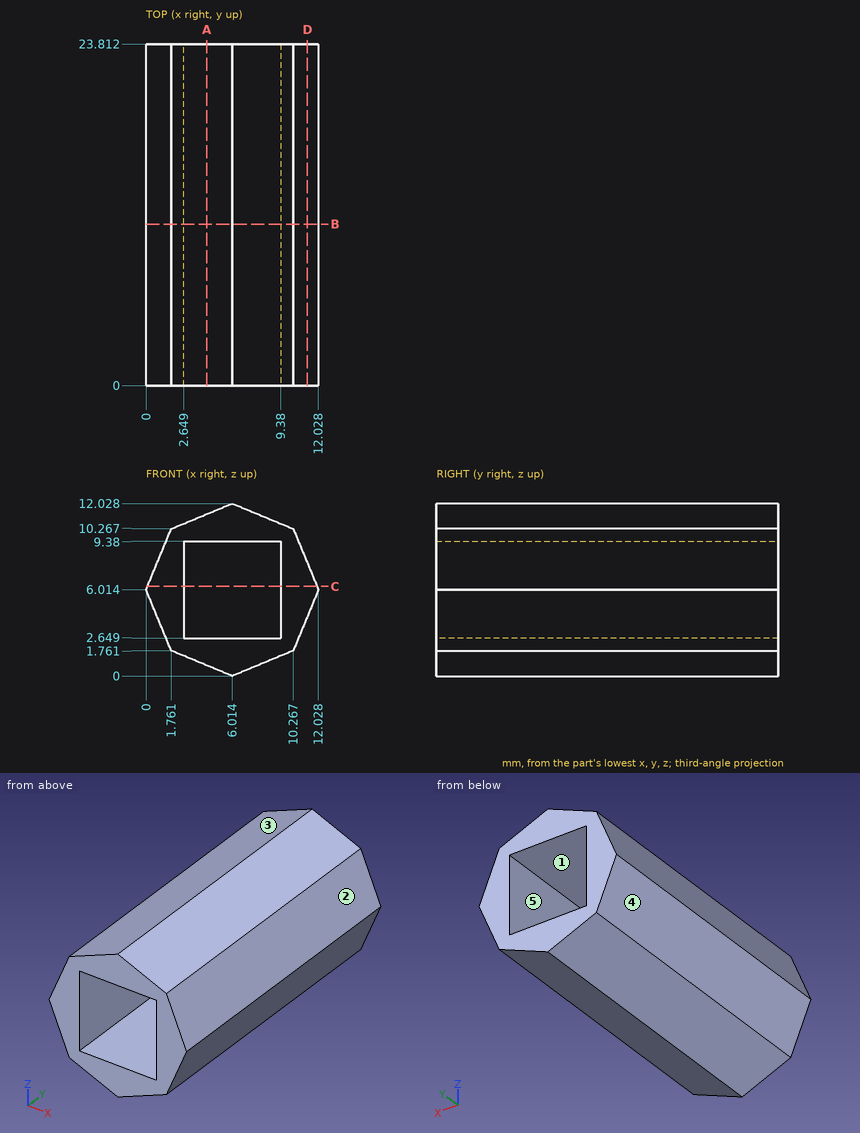
Print and shaded views of the part. All mm, measured from the part's lowest x, y and z. A direction names the side the tool comes from. Round coordinates to 2 decimals unless told otherwise and drop trailing zeros. Write each loop counter-clockwise with the first axis right and the second up, starting at its lowest first coordinate (ties: lowest second). Pieces come first, ordered by that corner, then holes. Notation, with made-up numbers: M 55,-20.75 L 80,-20.75 A10 ccw 80,-8.75 Z; hole C 38,40 d1. An arc over 180 degrees is marked long. Use a Markdown table: item, result. Add a question column.
1. Pull direction Z, two halves, no side cores. Call the marked faces 3, 4 and 5: released by +Z, released by -Z, zero draft, split by the parting line, or undercut.
2. Slice it at D-D on x = 11.25. Give the cut face in (y, z) (1 decimal).
3. Slice it at A-A on x = 4.25. Give the cut face in (y, z).
4. 3-axis set-ups, long thin cutter, end or side, ignore diameter. For the marked faces 1 and 2: which of +Z, -Z, +X, -X, +Y, -Y reach the whole face in a straight line?
5. Slice it at C-C on z = 6.25. Give the cut face in (x, y).
6. Drill centre lines: probe 1 along Z at (x, y) = (4.25, 10); probe 2 along Z at (x, y) = (5, 12.25); probe 3 along X at (y, z) = (9, 7). Where is each one in solid material? Low to high.
7. Flat gauge pin, fed straight in: P1, Ø6, axis at x = 9.5, y = 19.5, coming from the +Z side. Where does the tip first touch, or does it go through?
8. Slice it at B-B on y = 11.25. Give the cut face in (x, z) (1 decimal).
Reply:
| question | item | result |
|---|---|---|
| 1 | face 3 | released by +Z |
| 1 | face 4 | released by -Z |
| 1 | face 5 | undercut |
| 2 | outline | M 0,4.1 L 23.8,4.1 L 23.8,7.9 L 0,7.9 Z |
| 3 | outline | M 0,0.73 L 23.81,0.73 L 23.81,2.65 L 0,2.65 Z; M 0,9.38 L 23.81,9.38 L 23.81,11.3 L 0,11.3 Z |
| 4 | face 1 | +Y, -Y |
| 4 | face 2 | +Z, +X, +Y, -Y |
| 5 | outline | M 0.1,0 L 2.65,0 L 2.65,23.81 L 0.1,23.81 Z; M 9.38,0 L 11.93,0 L 11.93,23.81 L 9.38,23.81 Z |
| 6 | probe 1 | z = 0.73 to 2.65, 9.38 to 11.3 |
| 6 | probe 2 | z = 0.42 to 2.65, 9.38 to 11.61 |
| 6 | probe 3 | x = 0.41 to 2.65, 9.38 to 11.62 |
| 7 | P1 | stops at z = 11.83 |
| 8 | outline | M 0,6 L 1.8,1.8 L 6,0 L 10.3,1.8 L 12,6 L 10.3,10.3 L 6,12 L 1.8,10.3 Z; hole M 2.6,2.6 L 9.4,2.6 L 9.4,9.4 L 2.6,9.4 Z |
